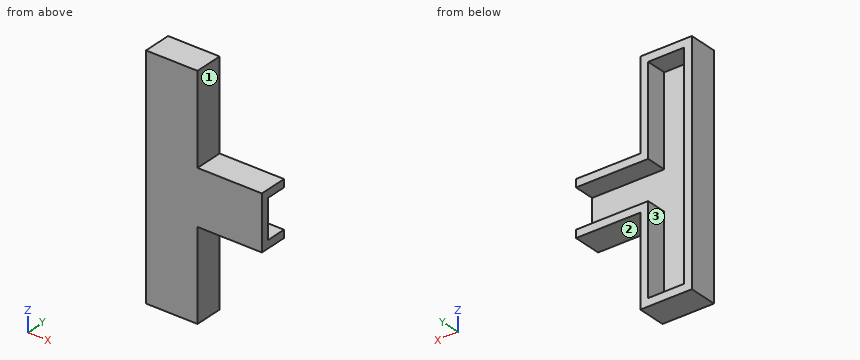
```python
from build123d import *

# Parameters (mm, degrees)
SKETCH1_W           = 16
SKETCH1_H           = 72
BOSS_EXTRUDE1_DEPTH = 2.4
SKETCH2_W           = 16
SKETCH2_H           = 72
SKETCH2_W_2         = 11.2
SKETCH2_H_2         = 67.2
BOSS_EXTRUDE2_DEPTH = 6.4
SKETCH3_W           = 12
SKETCH3_H           = 6.4
CUT_EXTRUDE1_DEPTH  = 4.8
BOSS_EXTRUDE3_DEPTH = 20


with BuildPart() as part:
    # Sketch1 → Boss-Extrude1 (new body)
    with BuildSketch(Plane(origin=(0, 0, 0), x_dir=(1, 0, 0), z_dir=(0, 1, 0))):
        with Locations((8, 36)):
            Rectangle(SKETCH1_W, SKETCH1_H)
    extrude(amount=BOSS_EXTRUDE1_DEPTH)

    # Sketch2 → Boss-Extrude2 (add)
    with BuildSketch(Plane(origin=(0, 2.4, 0), x_dir=(1, 0, 0), z_dir=(0, 1, 0))):
        with Locations((8, 36)):
            Rectangle(SKETCH2_W, SKETCH2_H)
        with Locations((8, 36)):
            Rectangle(SKETCH2_W_2, SKETCH2_H_2, mode=Mode.SUBTRACT)
    extrude(amount=BOSS_EXTRUDE2_DEPTH)

    # Sketch3 → Cut-Extrude1 (cut)
    with BuildSketch(Plane(origin=(16, 0, 0), x_dir=(0, 0, -1), z_dir=(1, 0, 0))):
        with Locations((36, 5.6)):
            Rectangle(SKETCH3_W, SKETCH3_H)
    extrude(amount=-CUT_EXTRUDE1_DEPTH, mode=Mode.SUBTRACT)

    # Sketch4 → Boss-Extrude3 (add)
    with BuildSketch(Plane(origin=(16, 0, 0), x_dir=(0, 0, -1), z_dir=(1, 0, 0))):
        Polygon((30, 2.4), (30, 8.8), (27.6, 8.8), (27.6, 0), (44.4, 0), (44.4, 8.8), (42, 8.8), (42, 2.4), align=None)
    extrude(amount=BOSS_EXTRUDE3_DEPTH)


solid = part.part
```
Geometry check sheet. Reference: the model listing, model coordinates, mm. Face numbers are marked on the shaded views. A direction names the side the tool comes from. Round coordinates to 2 decimals unless told otherwise and drop trailing zeros. Loops run counter-clockwise (first coordinate to the right, second up) from the corner with the lowest first, then second, coordinate; pieces in that order, holes last. Notation, with made-up numbers: (28, 31.5) - (52, 31.5) arc R27 ccw to (52, 59.5) - close; hole circle Ø1 at (-40, -19.5). An arc over 180 degrees is marked (long way). Write item = value, one per line. Start each with the question number.
1. Thickness scan on line 1 (Z direction, x = 14, y = 3.5); line 2 (X direction, y = 7.5, z = -18); line 3 (Z direction, x = 31, y = 3.5). Record the ranges inside material, lowest first.
2. Section check D-D on z = -31. Enter the section's corners in (x, y), then the cut area to 3 significant figures.
3. Set-up check for the marked faces 1, 2 and 3: record each of +Z, -Z, +X, -X, +Y, -Y from which the full face is reachable in a straight line by a thin tool's end or side.
4. Depth check by flat-ended pin: pin 1 (4.5 mm diameter, centred on y = 2.5, z = -61.5, fed in from +X); pin 2 (1.9 mm diameter, centred on y = 6, z = -40.5, fed in from +X); pin 3 (5 mm diameter, centred on x = 22, y = 6.5, fed in from -Z). Enter the tip coordinate at first touch or a pass-through.
5. Section check A-A on x = 26.5. Enter the section's corners in (y, z), then the cut area to 3 significant figures.
6. Section check B-B on z = -8. Enter the section's corners in (x, y).
7. Section check C-C on y = 8. Enter the section's corners in (x, z), then the cut area to 3 significant figures.
Working result:
q1.line_1 = -72 to -42, -30 to 0
q1.line_2 = 0 to 2.4, 13.6 to 16
q1.line_3 = -44.4 to -42, -30 to -27.6
q2.outline = (0, 0) - (36, 0) - (36, 2.4) - (2.4, 2.4) - (2.4, 8.8) - (0, 8.8) - close
q2.area = 102 mm^2
q3.face_1 = +Z, +X, +Y, -Y
q3.face_2 = -Z, +X, +Y, -Y
q3.face_3 = +Y
q4.pin_1 = 16
q4.pin_2 = 2.4
q4.pin_3 = -44.4
q5.outline = (0, -44.4) - (8.8, -44.4) - (8.8, -42) - (2.4, -42) - (2.4, -30) - (8.8, -30) - (8.8, -27.6) - (0, -27.6) - close
q5.area = 71.0 mm^2
q6.outline = (0, 0) - (16, 0) - (16, 8.8) - (13.6, 8.8) - (13.6, 2.4) - (2.4, 2.4) - (2.4, 8.8) - (0, 8.8) - close
q7.outline = (0, -72) - (16, -72) - (16, -44.4) - (36, -44.4) - (36, -42) - (13.6, -42) - (13.6, -69.6) - (2.4, -69.6) - (2.4, -2.4) - (13.6, -2.4) - (13.6, -30) - (36, -30) - (36, -27.6) - (16, -27.6) - (16, 0) - (0, 0) - close
q7.area = 467 mm^2
